Could you check a few things on this model? Use its own coordinates, in mm. Round coordinates to 2 decimals unless told otherwise and drop trailing zeros. Loops run counter-clockwise (first coordinate to the right, second up) from the corner with the lowest first, then second, coordinate; pieces in that order, holes last. Notation, with made-up numbers: (83, 75.25) - (94, 75.25) arc R21 ccw to (94, 81.25) - close; hole circle Ø6 at (21.5, 65). An arc over 180 degrees is marked (long way). Use one line per item in the form item = value.
```python
from build123d import *

# Parameters (mm, degrees)
SKETCH1_R           = 1.3462
SKETCH1_W           = 5.4034
SKETCH1_H           = 22.6066
SKETCH1_W_2         = 60.6932
SKETCH1_H_2         = 7.81
SKETCH1_W_3         = 15.431
SKETCH1_H_3         = 21.4039
SKETCH1_W_4         = 31.9679
SKETCH1_H_4         = 18.2371
SKETCH1_W_5         = 5.588
SKETCH1_H_5         = 33.5001
BOSS_EXTRUDE1_DEPTH = 3.048
SKETCH2_W           = 33.5789
SKETCH2_H           = 38.5801
CUT_EXTRUDE1_DEPTH  = 4.048
FILLET1_R           = 2.54
SKETCH3_R           = 1.524
CUT_EXTRUDE2_DEPTH  = 4.048
SKETCH4_W           = 43.3979
SKETCH4_H           = 3.81
CUT_EXTRUDE3_DEPTH  = 4.048
SKETCH5_W           = 12.7
SKETCH5_H           = 1.397
BOSS_EXTRUDE2_DEPTH = 3.048
SKETCH6_W           = 4.1917
SKETCH6_H           = 7.175
CUT_EXTRUDE4_DEPTH  = 4.048


with BuildPart() as part:
    # Sketch1 → Boss-Extrude1 (new body)
    with BuildSketch(Plane.XY):
        with BuildLine():
            Line((61.214907375, 24.068294304), (40.134807375, 24.068294304))
            Line((40.134807375, 24.068294304), (40.134807375, 8.658194304))
            Line((40.134807375, 8.658194304), (56.975007375, 8.658194304))
            Line((56.975007375, 8.658194304), (56.975007375, 4.997894304))
            Line((56.975007375, 4.997894304), (40.134807375, 4.997894304))
            Line((40.134807375, 4.997894304), (40.134807375, -9.121805696))
            Line((40.134807375, -9.121805696), (56.975007375, -9.121805696))
            Line((56.975007375, -9.121805696), (56.975007375, -12.628005696))
            Line((56.975007375, -12.628005696), (35.575007375, -12.628005696))
            Line((35.575007375, -12.628005696), (35.575007375, -28.627805696))
            Line((35.575007375, -28.627805696), (61.214907375, -28.627805696))
            Line((61.214907375, -28.627805696), (61.214907375, -32.613401529))
            ThreePointArc((61.214907375, -32.613401529), (60.108826144, -35.325305244), (57.405007375, -36.451005696))
            Line((57.405007375, -36.451005696), (38.714307375, -36.451005696))
            Line((38.714307375, -36.451005696), (28.474307375, -33.084405696))
            Line((28.474307375, -33.084405696), (-23.844892625, -33.084405696))
            Line((-23.844892625, -33.084405696), (-34.084892625, -36.451005696))
            ThreePointArc((-34.084892625, -36.451005696), (-36.778969461, -35.335082532), (-37.894892625, -32.641005696))
            Line((-37.894892625, -32.641005696), (-37.894892625, 26.697694304))
            ThreePointArc((-37.894892625, 26.697694304), (-36.778969461, 29.391771141), (-34.084892625, 30.507694304))
            Line((-34.084892625, 30.507694304), (57.404932375, 30.507694304))
            ThreePointArc((57.404932375, 30.507694304), (60.103884597, 29.386886916), (61.214907375, 26.683892153))
            Line((61.214907375, 26.683892153), (61.214907375, 24.068294304))
        make_face()
        with Locations((57.404932375, 26.697694304)):
            Circle(SKETCH1_R, mode=Mode.SUBTRACT)
        with Locations((57.405007375, -32.641005696)):
            Circle(SKETCH1_R, mode=Mode.SUBTRACT)
        with Locations((-34.084892625, -32.641005696)):
            Circle(SKETCH1_R, mode=Mode.SUBTRACT)
        with Locations((-34.084892625, 26.697694304)):
            Circle(SKETCH1_R, mode=Mode.SUBTRACT)
        with Locations((16.546707375, -19.663505696)):
            Rectangle(SKETCH1_W, SKETCH1_H, mode=Mode.SUBTRACT)
        with Locations((1.341707375, 21.991994304)):
            Rectangle(SKETCH1_W_2, SKETCH1_H_2, mode=Mode.SUBTRACT)
        with Locations((25.156507375, 5.270444304)):
            Rectangle(SKETCH1_W_3, SKETCH1_H_3, mode=Mode.SUBTRACT)
        with Locations((-5.654942625, 1.475544304)):
            Rectangle(SKETCH1_W_4, SKETCH1_H_4, mode=Mode.SUBTRACT)
        with Locations((-26.210892625, -6.948855696)):
            Rectangle(SKETCH1_W_5, SKETCH1_H_5, mode=Mode.SUBTRACT)
    extrude(amount=BOSS_EXTRUDE1_DEPTH)

    # Sketch2 → Cut-Extrude1 (cut, through all)
    with BuildSketch(Plane.XY.offset(3.048)):
        with Locations((-4.849442625, -6.948855696)):
            Rectangle(SKETCH2_W, SKETCH2_H)
    extrude(amount=-CUT_EXTRUDE1_DEPTH, mode=Mode.SUBTRACT)

    # Fillet1
    fillet1_edges = [part.edges().sort_by_distance(p)[0] for p in [
        (-21.638892625, -26.238905696, 1.524),
        (11.940007375, 12.341194304, 1.524),
        (11.940007375, -26.238905696, 1.524),
        (-21.638892625, 12.341194304, 1.524),
    ]]
    fillet(fillet1_edges, radius=FILLET1_R)

    # Sketch3 → Cut-Extrude2 (cut, through all)
    with BuildSketch(Plane.XY.offset(3.048)):
        with Locations((-34.084892625, 26.697694304)):
            Circle(SKETCH3_R)
        with Locations((57.404932375, 26.697694304)):
            Circle(SKETCH3_R)
        with Locations((57.405007375, -32.641005696)):
            Circle(SKETCH3_R)
        with Locations((-34.084892625, -32.641005696)):
            Circle(SKETCH3_R)
    extrude(amount=-CUT_EXTRUDE2_DEPTH, mode=Mode.SUBTRACT)

    # Sketch4 → Cut-Extrude3 (cut, through all)
    with BuildSketch(Plane.XY.offset(3.048)):
        with Locations((-7.305942625, 16.181994304)):
            Rectangle(SKETCH4_W, SKETCH4_H)
    extrude(amount=-CUT_EXTRUDE3_DEPTH, mode=Mode.SUBTRACT)

    # Sketch5 → Boss-Extrude2 (add)
    with BuildSketch(Plane.XY.offset(3.048)):
        with Locations((49.149907375, 23.369794304)):
            Rectangle(SKETCH5_W, SKETCH5_H)
    extrude(amount=-BOSS_EXTRUDE2_DEPTH)

    # Sketch6 → Cut-Extrude4 (cut, through all)
    with BuildSketch(Plane.XY.offset(3.048)):
        with Locations((33.784157375, 21.674494304)):
            Rectangle(SKETCH6_W, SKETCH6_H)
    extrude(amount=-CUT_EXTRUDE4_DEPTH, mode=Mode.SUBTRACT)


solid = part.part
```
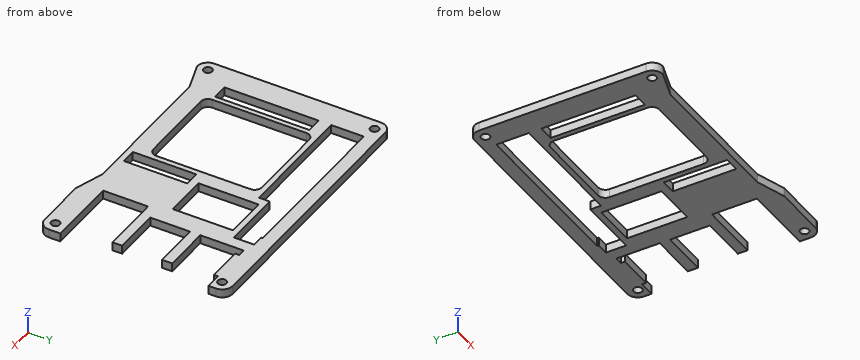
1. For P1, Ø0.9, axis at x = -1, z = 1.5, coming from the -Y side; P2, Ø1.5, axis at y = -11, z = 2, coming from the +X side (3 decimals); P3, Ø1.5, axis at x = 29, z = 2, coming from the -Y side, each with a flat end and sliding along its axis, tell me the tip position at first contact or that it passes through.
Solution:
P1 = -33.08
P2 = 56.975
P3 = -33.5
2. If we section it at D-D, the plane x = -27: Write out the boundary of the cut face in (y, z), plus the area to 3 significant figures.
Solution:
outline = (-34.12, 0) - (-23.7, 0) - (-23.7, 3.05) - (-34.12, 3.05) - close; (9.8, 0) - (14.28, 0) - (14.28, 3.05) - (9.8, 3.05) - close; (25.9, 0) - (30.51, 0) - (30.51, 3.05) - (25.9, 3.05) - close
area = 59.5 mm^2
3. If we section it at A-A, the plane x = 16: Write out the boundary of the cut face in (y, z), plus the area to 3 significant figures.
Solution:
outline = (-33.08, 0) - (-30.97, 0) - (-30.97, 3.05) - (-33.08, 3.05) - close; (-8.36, 0) - (18.09, 0) - (18.09, 3.05) - (-8.36, 3.05) - close; (25.9, 0) - (30.51, 0) - (30.51, 3.05) - (25.9, 3.05) - close
area = 101 mm^2
4. If we section it at B-B, the plane y = 1.5: Write out the boundary of the cut face in (x, z).
Solution:
outline = (-37.89, 0) - (-29, 0) - (-29, 3.05) - (-37.89, 3.05) - close; (-23.42, 0) - (-21.64, 0) - (-21.64, 3.05) - (-23.42, 3.05) - close; (11.94, 0) - (17.44, 0) - (17.44, 3.05) - (11.94, 3.05) - close; (32.87, 0) - (40.13, 0) - (40.13, 3.05) - (32.87, 3.05) - close
5. Please list where these lines run through material, in increasing order: line 1 along X through (y, z) = (-9, 1.45) (3 decimals); line 2 along X through (y, z) = (-11, 0.65) (3 decimals); line 3 along Y through (x, z) = (-11, 2.4).
Solution:
line_1 = -37.895 to -29.005, -23.417 to -21.639, 11.94 to 13.845, 19.248 to 40.135
line_2 = -37.895 to -29.005, -23.417 to -21.639, 11.94 to 13.845, 19.248 to 56.975
line_3 = -33.08 to -26.24, 12.34 to 14.28, 25.9 to 30.51
6. If we section it at C-C, the plane z = 0.75: Count the separate pieces of the cut face and the enclosed holes in it, plus the area to 3 significant figures.
Solution:
separate_pieces = 1
enclosed_holes = 9
area = 2,740 mm^2
